Part model, mm, in its own coordinate system. A direction names the side the tool comes from. Coordinates: 2 decimals unless noted, no trailing zeros. Order: outer loops, then holes, each group sorted by start corner. A loop starts at its lowest first (then second) coordinate and runs counter-clockwise, first axis right, second up.
Autodesk Inventor part; units mm, degrees
ref_plane "Work Plane1" through (0, 0, -7) normal (0, 0, -1) x (-1, 0, 0)
ref_plane "YZ Plane" through (0, 0, 0) normal (1, 0, 0) x (0, 1, 0)
ref_plane "XZ Plane" through (0, 0, 0) normal (0, 1, 0) x (-1, 0, 0)
sketch "Sketch1" plane through (0, 0, 0) normal (0, 0, 1) x (1, 0, 0)
  circle A0 centre (0, 0) radius 5.5
  dimension "d0" = 11
extrude "Extrusion1" add sketch "Sketch1" along normal blind 7
sketch "Sketch2" plane through (0, 0, 7) normal (0, 0, 1) x (1, 0, 0)
  circle A0 centre (0, 0) radius 3.5
  dimension "d3" = 7
extrude "Extrusion2" add sketch "Sketch2" along normal blind 1
sketch "Sketch4" plane through (0, 0, 8) normal (0, 0, 1) x (1, 0, 0)
  circle A0 centre (0, 0) radius 1.5
  dimension "d7" = 3
hole "Hole1" at (0, 0, 8) direction (0, 0, -1) diameter 3 end through all
fillet "Fillet1" radius 0.3 1 edges at (-3.5, 0, 8)
fillet "Fillet2" radius 0.3 1 edges at (-5.5, 0, 7)
sketch "Sketch5" plane through (0, 0, 0) normal (0, 0, -1) x (-1, 0, 0)
  circle A0 centre (0, 0) radius 1.5
  circle A1 centre (0, 0) radius 3
  dimension "d17" = 6
ref_plane "Work Plane1" through (0, 0, -7) normal (0, 0, -1) x (-1, 0, 0)
sketch "Sketch6" plane through (0, 0, -7) normal (0, 0, -1) x (-1, 0, 0)
  circle A0 centre (0, 0) radius 2.5
  dimension "d19" = 5
loft "Loft1" add profiles "Sketch6", "Sketch5" contours all / A0 | A1
sketch "Sketch7" plane through (0, 0, 0) normal (0, 0, 1) x (1, 0, 0)
  point P0 (0, 0)
  point P1 (0, 0)
hole "Hole2" at (0, 0, 0) at (0, 0, 0) direction (0, 0, -1) diameter 3 end through all
thread "Thread1"
properties part number "Banana Hembra"
Q1. Which spindle directions (+Z, -Z, +X, -X, +Y, -Y) get a long thin tool onto all of the face, cutting with end or side? Do faces 1 (the face through (3.233, 1.341, 7.345)), 2 (the face through (0.7, 1.5, 8)). Say none if no direction does.
Results list:
face 1: +Z
face 2: +Z, +X, -X, +Y, -Y
Q2. Mould opens along X. For faces 3 (the face through (2.03, -1.86, -3.45)), 4 (the face through (-0.07, 1.5, 0.39)), 5 (the face through (2.4, -2.4, 0)) say: pulls with the +X half, pulls with the -X half, needs draft (parallel to the pull), parting line crosses it, or undercut.
Results list:
face 3: parting line crosses it
face 4: undercut
face 5: needs draft
Q3. Cut at B-B on z = 3.75. Write the cut outline in (x, y), and give its area (3 significant figures).
Results list:
outline: circle Ø11 at (0, 0); hole circle Ø3 at (0, 0)
area: 88.0 mm2
Q4. Cut at A-A on x = 0. Write the cut outline in (y, z).
Results list:
outline: (-5.5, 0) - (-3, 0) - (-2.5, -7) - (-1.5, -7) - (-1.5, 8) - (-3.2, 8) arc R0.3 ccw to (-3.5, 7.7) - (-3.5, 7) - (-5.2, 7) arc R0.3 ccw to (-5.5, 6.7) - close; (1.5, -7) - (2.5, -7) - (3, 0) - (5.5, 0) - (5.5, 6.7) arc R0.3 ccw to (5.2, 7) - (3.5, 7) - (3.5, 7.7) arc R0.3 ccw to (3.2, 8) - (1.5, 8) - close
Q5. Pin check, flat tips, straight feed: pin 1 Ø6 at (x, z) = (-3, -5) entering from +Y; pin 2 Ø2 at (x, z) = (-0.5, -4) entering from +Y; pin 3 Ø4 at (x, z) = (2.5, -5) entering from +Y; pin 4 Ø6 at (y, z) = (0.5, 3.5) entering from -X. Stop position of each tip, or through.
Results list:
pin 1: stops at y = 2.72
pin 2: stops at y = 2.78
pin 3: stops at y = 2.62
pin 4: stops at x = -5.5
Q6. Wall check: line 1 along Y through (x, z) = (0, 3.5); line 2 along Z through (x, y) = (3.75, -1.5); line 3 along X through (y, z) = (0.5, -0.5). Give the ranges that are in metal, low to high.
Results list:
line 1: y = -5.5 to -1.5, 1.5 to 5.5
line 2: z = 0 to 7
line 3: x = -2.92 to -1.41, 1.41 to 2.92
